For this review, take the finished solid that the model builds, in its own axes (mm). Face numbers are marked on the shaded views. A direction names the side the tool comes from. Coordinates: 2 decimals unless noted, no trailing zeros. Loops run counter-clockwise (first coordinate to the right, second up) from the corner with the lowest first, then second, coordinate; pieces in that order, holes last.
1. To check wall thickness, follow probe 1 along Y at (x, z) = (21, -14); probe 2 along X at (y, z) = (0, -13); probe 3 along Y at (x, z) = (1.5, -16). State the ranges of each line that lie inside material, in increasing order.
2. Clearance check with flat-ended pins moving along their axes: P1, Ø1, axis at y = -17, z = 10.5, coming from the -X side; P2, Ø3, axis at y = 19, z = -8.5, coming from the +X side; P3, Ø18.5, axis at x = 0, y = 44.45, coming from the +Z side; P4, Ø12, axis at y = -50.5, z = -8.5, coming from the +X side. State where each tip first meets the part, or that it passes through.
3. Take a section at C-C, the plane z = 15.5. State the section outline as (x, y) points, then the cut area to 3 significant figures.
4. Mouldability with a two-part tool opening along X and no side actions: class the marked faces 4, 5 and 6 as pulls with the +X half, pulls with the -X half, needs draft (parallel to the pull), parting line crosses it, or undercut.
5. Take a section at A-A, the plane y = 0. State the section outline as (x, z) points (3 decimals), then the cut area to 3 significant figures.
6. Machinability: for the marked faces 1, 2 and 3, which of the approach directions +Z, -Z, +X, -X, +Y, -Y give a long, thin tool a straight path to every point of the face, cutting with its end or side? Answer none if there is none.
7. Take a section at B-B, the plane x = 0. State the section outline as (y, z) points (3 decimals).
8. Take a section at D-D, the plane z = -1. State the section outline as (x, y) points (3 decimals), then the cut area to 3 significant figures.
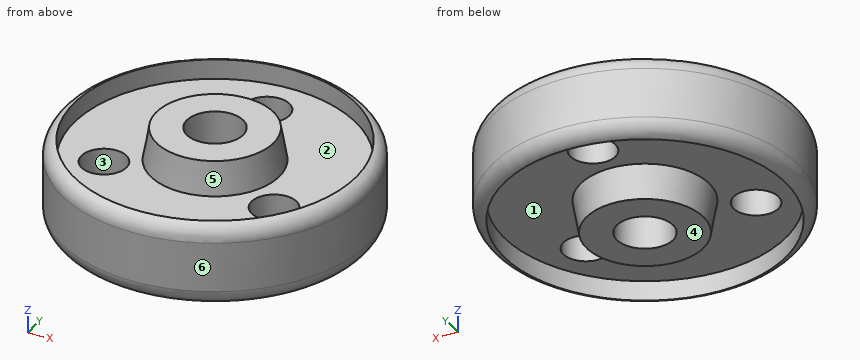
```python
from build123d import *

# Parameters (mm, degrees)
SKETCH2_R          = 10.16
CUT_EXTRUDE2_DEPTH = 254
CIRPATTERN1_COUNT  = 3
FILLET1_R          = 7.62


with BuildPart() as part:
    # Sketch1 → Revolve1 (revolve)
    with BuildSketch(Plane(origin=(0, 0, 0), x_dir=(0, 0, -1), z_dir=(1, 0, 0)), mode=Mode.PRIVATE) as revolve1_sk:
        Polygon((-24.384, 12.7), (-24.384, 26.416), (-9.525, 29.036042606), (-9.525, 63.5), (-18.542, 63.5), (-18.542, 68.834), (18.542, 68.834), (18.542, 63.5), (9.525, 63.5), (9.525, 29.036042606), (24.384, 26.416), (24.384, 12.7), align=None)
    revolve(revolve1_sk.sketch.rotate(Axis((0, 0, 0), (0, 0, -1)), 180), axis=Axis((0, 0, 0), (0, 0, -1)))

    # Sketch2 → Cut-Extrude2 (cut, symmetric)
    with BuildSketch(Plane.XY):
        with Locations(Location((0, 44.45, 0), (0, 0, 90))):
            Circle(SKETCH2_R)
    cut_extrude2 = extrude(amount=CUT_EXTRUDE2_DEPTH, both=True, mode=Mode.SUBTRACT)

    # CirPattern1: Cut-Extrude2 ×3 about axis
    cirpattern1_axis = Axis((0, 0, 0), (0, 0, 1))
    for i in range(1, CIRPATTERN1_COUNT):
        add(cut_extrude2.rotate(cirpattern1_axis, i * 360 / CIRPATTERN1_COUNT), mode=Mode.SUBTRACT)

    # Fillet1
    # the kernel refuses this fillet: 7.62 mm, written as the material it takes off along each edge
    with BuildSketch(Plane(origin=(0, 0, 18.542), x_dir=(0, -1, 0), z_dir=(1, 0, 0))) as fillet1_piece_1:
        with BuildLine():
            CenterArc((61.214, 7.269016715), FILLET1_R, 287.457603124, 72.542396876)
            Line((68.834, 7.269016715), (68.9864, 7.269016715))
            Line((68.9864, 7.269016715), (68.9864, 0))
            Line((68.9864, 0), (68.834, -0.1524))
            ThreePointArc((68.834, -0.1524), (66.167, -0.1524), (63.54572, -0.145380334))
            Line((63.54572, -0.145380334), (63.5, 0))
        make_face()
    revolve(axis=Axis((0, 0, 18.542), (0, 0, -1)), mode=Mode.SUBTRACT)
    with BuildSketch(Plane(origin=(0, 0, -18.542), x_dir=(0, -1, 0), z_dir=(1, 0, 0))) as fillet1_piece_2:
        with BuildLine():
            CenterArc((61.214, -7.269016715), FILLET1_R, 0, 72.542396876)
            Line((63.5, 0), (63.54572, 0.145380334))
            ThreePointArc((63.54572, 0.145380334), (66.167, 0.1524), (68.834, 0.1524))
            Line((68.834, 0.1524), (68.9864, 0))
            Line((68.9864, 0), (68.9864, -7.269016715))
            Line((68.9864, -7.269016715), (68.834, -7.269016715))
        make_face()
    revolve(axis=Axis((0, 0, -18.542), (0, 0, -1)), mode=Mode.SUBTRACT)


solid = part.part
```
Results list:
1. probe 1: y = -65.02 to -59.93, -18.89 to 18.89, 59.93 to 65.02
1. probe 2: x = -68.64 to -63.5, -28.42 to -12.7, 12.7 to 28.42, 63.5 to 68.64
1. probe 3: y = -67.17 to -63.48, -27.85 to -12.61, 12.61 to 27.85, 63.48 to 67.17
2. P1: stops at x = -66.83
2. P2: stops at x = 66.57
2. P3: passes through
2. P4: stops at x = 52.52
3. outline: circle Ø135.11 at (0, 0); circle Ø55.96 at (0, 0); hole circle Ø127 at (0, 0); hole circle Ø25.4 at (0, 0)
3. area: 3,620 mm2
4. face 4: needs draft
4. face 5: undercut
4. face 6: parting line crosses it
5. outline: (-68.834, -11.273) arc R7.62 ccw to (-63.5, -18.542) - (-63.5, -9.525) - (-29.036, -9.525) - (-26.416, -24.384) - (-12.7, -24.384) - (-12.7, 24.384) - (-26.416, 24.384) - (-29.036, 9.525) - (-63.5, 9.525) - (-63.5, 18.542) arc R7.62 ccw to (-68.834, 11.273) - close; (12.7, -24.384) - (26.416, -24.384) - (29.036, -9.525) - (63.5, -9.525) - (63.5, -18.542) arc R7.62 ccw to (68.834, -11.273) - (68.834, 11.273) arc R7.62 ccw to (63.5, 18.542) - (63.5, 9.525) - (29.036, 9.525) - (26.416, 24.384) - (12.7, 24.384) - close
5. area: 3,180 mm2
6. face 1: -Z
6. face 2: +Z
6. face 3: +Z, -Z
7. outline: (-68.834, -11.273) arc R7.62 ccw to (-63.5, -18.542) - (-63.5, -9.525) - (-29.036, -9.525) - (-26.416, -24.384) - (-12.7, -24.384) - (-12.7, 24.384) - (-26.416, 24.384) - (-29.036, 9.525) - (-63.5, 9.525) - (-63.5, 18.542) arc R7.62 ccw to (-68.834, 11.273) - close; (12.7, -24.384) - (26.416, -24.384) - (29.036, -9.525) - (34.29, -9.525) - (34.29, 9.525) - (29.036, 9.525) - (26.416, 24.384) - (12.7, 24.384) - close; (54.61, -9.525) - (63.5, -9.525) - (63.5, -18.542) arc R7.62 ccw to (68.834, -11.273) - (68.834, 11.273) arc R7.62 ccw to (63.5, 18.542) - (63.5, 9.525) - (54.61, 9.525) - close
8. outline: circle Ø137.668 at (0, 0); hole circle Ø20.32 at (-38.495, -22.225); hole circle Ø25.4 at (0, 0); hole circle Ø20.32 at (0, 44.45); hole circle Ø20.32 at (38.495, -22.225)
8. area: 13,400 mm2
